Input: part model. Units: mm. Frame: model coordinates. Face numbers are marked on the shaded views. A direction names the side the tool comes from. Give positions to 0.01 mm unless a question says otherwise; leave off trailing zeros. Loops run counter-clockwise (first coordinate to the right, second up) from the corner with the lowest first, then second, coordinate; pieces in that order, holes last. Notation, with made-up numbers: (-8.75, 31) - (35.25, 31) arc R16 cw to (35.25, 39) - close; hole circle Ø5 at (-35.5, -13). An arc over 180 degrees is marked (long way). Answer as a JSON object with one key per item and string values. Group by question number.
(1) Section query C-C (x = 105). Return loops of the section in (y, z).
(2) Material intervals for L1, parallel to Z at x = 72, y = 0; L2, parallel to Y at x = 61, z = 0; L3, parallel to Y at x = 48, z = -12.5, sorted ascending.
(3) Section query B-B (y = 6.5). Return loops of the section in (x, z).
(4) Pin query (flat end, axial travel): P1, Ø1, axis at x = 60, z = -20, coming from the -Y side; P2, Ø4, axis at x = 57.5, y = -37.5, coming from the +Z side; P3, Ø4, axis at x = 133.5, y = 38.5, coming from the -Z side. Return the tip coordinate at first contact, or that it passes through.
(5) Mould query, pull axis Z, two halves, no side actions, for the marked faces 3 and 4. Classes: +Z half, -Z half, draft (parallel to the pull), parting line (faces both ways), or undercut.
(6) Access query for the marked faces 1 and 2. Directions: +Z, -Z, +X, -X, +Y, -Y. A direction counts if a zero-diameter tool reaches every point of the face in a straight line with its end or side. Return the directions, or none.
(7) Section query A-A (z = 0). Return loops of the section in (x, y), plus the area to 3 significant figures.
(8) Section query D-D (x = 160). Return loops of the section in (y, z), plus the area to 3 significant figures.
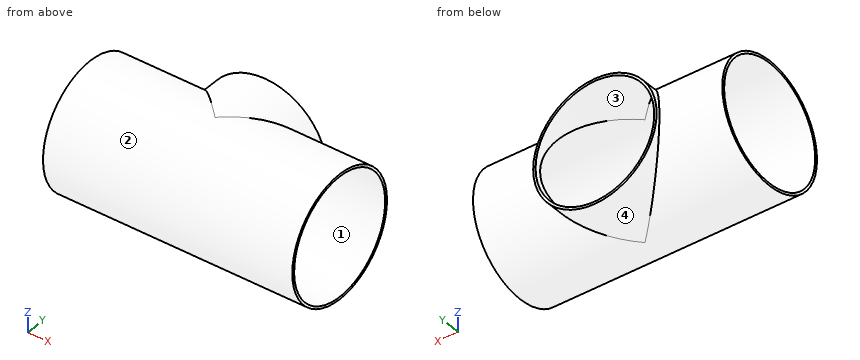
```python
from build123d import *

# Parameters (mm, degrees)
SKETCH1_W                  = 210
SKETCH1_H                  = 52
SKETCH2_W                  = 52
SKETCH2_H                  = 55
M90_CLEARANCE_HOLE1_D      = 100
M90_CLEARANCE_HOLE2_REACH  = 243.357
M90_CLEARANCE_HOLE2_BORE_R = 50


with BuildPart() as part:
    # Sketch1 → Revolve1 (revolve)
    with BuildSketch(Plane.XY, mode=Mode.PRIVATE) as revolve1_sk:
        with Locations((105, 26)):
            Rectangle(SKETCH1_W, SKETCH1_H)
    revolve(revolve1_sk.sketch.rotate(Axis((0, 0, 0), (1, 0, 0)), 270), axis=Axis((0, 0, 0), (1, 0, 0)))

    # Sketch2 → Revolve2 (revolve)
    with BuildSketch(Plane.XY, mode=Mode.PRIVATE) as revolve2_sk:
        with Locations((79, 27.5)):
            Rectangle(SKETCH2_W, SKETCH2_H)
    revolve(revolve2_sk.sketch.rotate(Axis((105, 0, 0), (0, 1, 0)), 90), axis=Axis((105, 0, 0), (0, 1, 0)))

    # M90 Clearance Hole1 (through all)
    with Locations(Plane(origin=(210, 0, 0), x_dir=(0, 0, -1), z_dir=(1, 0, 0))):
        with Locations((0, 0)):
            Hole(M90_CLEARANCE_HOLE1_D / 2)

    # M90 Clearance Hole2 bore → M90 Clearance Hole2 (cut, up to next)
    with BuildSketch(Plane(origin=(0, 55, 0), x_dir=(1, 0, 0), z_dir=(0, 1, 0)), mode=Mode.PRIVATE) as m90_clearance_hole2_sk1:
        with Locations((105, 0)):
            Circle(M90_CLEARANCE_HOLE2_BORE_R)
    m90_clearance_hole2_tool1 = extrude(m90_clearance_hole2_sk1.sketch, amount=-M90_CLEARANCE_HOLE2_REACH, mode=Mode.PRIVATE) & part.part
    add(m90_clearance_hole2_tool1.solids().sort_by_distance((105, 55, 0))[0], mode=Mode.SUBTRACT)


solid = part.part
```
Recorded:
{
 "1": {"outline": "(0, -52) - (55, -52) - (55, -50) - (0, -50) arc R50 cw to (0, 50) - (55, 50) - (55, 52) - (0, 52) arc R52 ccw to start"},
 "2": {"L1": "z = -52 to -50, 50 to 52", "L2": "y = -52 to -50", "L3": "y = -50.48 to -48.41, 48.41 to 50.48"},
 "3": {"outline": "(0, -51.59) - (98.5, -51.59) arc R52 ccw to (111.5, -51.59) - (210, -51.59) - (210, -49.58) - (111.5, -49.58) arc R50 cw to (98.5, -49.58) - (0, -49.58) - close; (0, 49.58) - (98.5, 49.58) arc R50 cw to (111.5, 49.58) - (210, 49.58) - (210, 51.59) - (111.5, 51.59) arc R52 ccw to (98.5, 51.59) - (0, 51.59) - close"},
 "4": {"P1": "stops at y = -48.21", "P2": "stops at z = 38", "P3": "stops at z = -44.74"},
 "5": {"face 3": "undercut", "face 4": "parting line"},
 "6": {"face 1": "+X, -X", "face 2": "none"},
 "7": {"outline": "(0, -52) - (210, -52) - (210, -50) - (0, -50) - close; (0, 50) - (55, 50) - (55, 55) - (53, 55) - (53, 52) - (0, 52) - close; (155, 50) - (210, 50) - (210, 52) - (157, 52) - (157, 55) - (155, 55) - close", "area": "652 mm^2"},
 "8": {"outline": "circle Ø104 at (0, 0); hole circle Ø100 at (0, 0)", "area": "641 mm^2"}
}
